Here's how the part is built. I have some questions about the finished solid (model axes, mm). A direction names the side the tool comes from. Coordinates: 2 decimals unless noted, no trailing zeros. Write each loop counter-clockwise with the first axis right and the second up, starting at its lowest first coordinate (ties: lowest second). Pieces come first, ordered by that corner, then holes. Notation, with made-up numbers: (84, 31.5) -> (95, 31.5) arc R23 cw to (95, 53.5) -> close; hole circle Ø5 at (-30.75, 50.25). An arc over 180 degrees is marked (long way). Answer in a Markdown table with one row per item. Add a question column.
from build123d import *

# Parameters (mm, degrees)
CROQUIS1_R                   = 50
SALIENTE_EXTRUIR1_DEPTH      = 120
CORTAR_EXTRUIR1_REACH        = 141.284
CROQUIS2_R                   = 45
SALIENTE_EXTRUIR2_REACH      = 141.284
SALIENTE_EXTRUIR2_END_RADIUS = 45
CROQUIS4_W                   = 47
CROQUIS4_H                   = 42
CROQUIS5_W                   = 47
CROQUIS5_H                   = 42
CORTAR_EXTRUIR2_DEPTH        = 14
CORTAR_EXTRUIR3_REACH        = 141.284


with BuildPart() as part:
    # Croquis1 → Saliente-Extruir1 (new body)
    with BuildSketch(Plane(origin=(0, 0, 0), x_dir=(1, 0, 0), z_dir=(0, 1, 0))):
        with Locations(Location((0, 0, 0), (0, 0, 270))):
            Circle(CROQUIS1_R)
    extrude(amount=SALIENTE_EXTRUIR1_DEPTH)

    # Croquis2 → Cortar-Extruir1 (cut, up to next)
    with BuildSketch(Plane(origin=(0, 120, 0), x_dir=(1, 0, 0), z_dir=(0, 1, 0)), mode=Mode.PRIVATE) as cortar_extruir1_sk1:
        with Locations(Location((0, 0, 0), (0, 0, 270))):
            Circle(CROQUIS2_R)
    cortar_extruir1_tool1 = extrude(cortar_extruir1_sk1.sketch, amount=-CORTAR_EXTRUIR1_REACH, mode=Mode.PRIVATE) & part.part
    add(cortar_extruir1_tool1.solids().sort_by_distance((0, 120, 0))[0], mode=Mode.SUBTRACT)

    # Saliente-Extruir2: up to this cylinder (the profile starts inside it)
    saliente_extruir2_end = Plane(origin=(0, 63, 0), z_dir=(0, 1, 0)) * Cylinder(SALIENTE_EXTRUIR2_END_RADIUS, 373.568, mode=Mode.PRIVATE)
    # Croquis4 → Saliente-Extruir2 (add, up to the surface)
    with BuildSketch(Plane.XY, mode=Mode.PRIVATE) as saliente_extruir2_sk1:
        with Locations((14.5, 63)):
            Rectangle(CROQUIS4_W, CROQUIS4_H)
    saliente_extruir2_tool1 = extrude(saliente_extruir2_sk1.sketch, amount=-SALIENTE_EXTRUIR2_REACH, mode=Mode.PRIVATE) & saliente_extruir2_end
    add(saliente_extruir2_tool1.solids().sort_by_distance((14.5, 63, 0))[0])

    # Croquis5 → Cortar-Extruir2 (cut)
    with BuildSketch(Plane.XY):
        with Locations((14.5, 63)):
            Rectangle(CROQUIS5_W, CROQUIS5_H)
    extrude(amount=-CORTAR_EXTRUIR2_DEPTH, mode=Mode.SUBTRACT)

    # Croquis7 → Cortar-Extruir3 (cut, up to next)
    with BuildSketch(Plane(origin=(0, 120, 0), x_dir=(1, 0, 0), z_dir=(0, 1, 0)), mode=Mode.PRIVATE) as cortar_extruir3_sk1:
        with BuildLine():
            Line((-9, -44.09081537), (-9, -49.183330509))
            ThreePointArc((-9, -49.183330509), (16.72918014, -47.118303576), (38, -32.496153619))
            Line((38, -32.496153619), (38, -24.103941586))
            ThreePointArc((38, -24.103941586), (17.61018969, -41.41112434), (-9, -44.09081537))
        make_face()
    cortar_extruir3_tool1 = extrude(cortar_extruir3_sk1.sketch, amount=-CORTAR_EXTRUIR3_REACH, mode=Mode.PRIVATE) & part.part
    add(cortar_extruir3_tool1.solids().sort_by_distance((16.242492, 120, 42.000337))[0], mode=Mode.SUBTRACT)


solid = part.part
Q1. I'm going to push flat-ended pins straight in: P1, Ø4, axis at x = 27, y = 50.5, coming from the +Z side; P2, Ø6, axis at y = 75, z = 27, coming from the -X side; P3, Ø3, axis at y = 70, z = -17, coming from the +X side; P4, Ø25, axis at x = 19.5, z = -31.5, coming from the -Y side. Where does each tip first touch, or does it pass through?
Q2. For faces 5 (the flat face through (-9, 63, -29)), 6 (the flat face through (-9, 61, 47)), 7 (the flat face through (14, 42, -29)), 8 (the flat face through (38, 61, 28)), 9 (the flat face through (14, 84, -29)), which set-ups out of +Z, -Z, +X, -X, +Y, -Y let a thin tool reach every point of the face, with its end or its side?
Q3. If we mould it in two halves opening along Z, with no side actions, what happens to faces 1 (the cylindrical face through (-14.99, 59.16, -47.7)), 2 (the flat face through (38, 63, -19)), 3 (the flat face through (14, 63, -14)), 4 (the flat face through (-7, 0, -45))? For each: pulls with the +Z half, pulls with the -Z half, needs draft (parallel to the pull), parting line crosses it, or undercut.
Q4. Imagine slicing it at D-D on x = -20. Please give me the cut outline in (y, z), plus the area to 3 significant figures.
Q5. Imagine slicing it at A-A on z = 0. Please give me the cut outline in (x, y), plus the area to 3 significant figures.
Q6. Imagine slicing it at C-C on y = 49. Please give me the cut outline in (x, z).
Q7. I need wall thicknesses on line 1 (X direction, y = 59.5, z = 0); line 2 (Z direction, x = 0, y = 39.5); line 3 (Z direction, x = 0, y = 70). Which ranges of each line are inside material? Lowest first, please. Write a range as [from, to].
Q8. Imagine slicing it at B-B on x = 0. Please give me the cut outline in (y, z).
Result sheet:
| question | item | result |
|---|---|---|
| 1 | P1 | stops at z = -14 |
| 1 | P2 | stops at x = -43.86 |
| 1 | P3 | stops at x = 47.54 |
| 1 | P4 | stops at y = 0 |
| 2 | face 5 | +Y, -Y |
| 2 | face 6 | +Z, +X, +Y, -Y |
| 2 | face 7 | +Z, -Y |
| 2 | face 8 | +Z, +Y, -Y |
| 2 | face 9 | +Z, +Y |
| 3 | face 1 | parting line crosses it |
| 3 | face 2 | undercut |
| 3 | face 3 | pulls with the +Z half |
| 3 | face 4 | needs draft |
| 4 | outline | (0, -45.83) -> (120, -45.83) -> (120, -40.31) -> (0, -40.31) -> close; (0, 40.31) -> (120, 40.31) -> (120, 45.83) -> (0, 45.83) -> close |
| 4 | area | 1,320 mm^2 |
| 5 | outline | (-50, 0) -> (-45, 0) -> (-45, 120) -> (-50, 120) -> close; (45, 0) -> (50, 0) -> (50, 120) -> (45, 120) -> close |
| 5 | area | 1,200 mm^2 |
| 6 | outline | (-9, -44.09) arc R45 cw to (-9, 44.09) -> (-9, 49.18) arc R50 ccw (long way) to (38, 32.5) -> (38, 24.1) arc R45 cw to (38, -24.1) -> (38, -14) -> (-9, -14) -> close |
| 7 | line 1 | x = [-50, -45], [45, 50] |
| 7 | line 2 | z = [-50, -45] |
| 7 | line 3 | z = [-50, -14] |
| 8 | outline | (0, -50) -> (120, -50) -> (120, -45) -> (84, -45) -> (84, -14) -> (42, -14) -> (42, -45) -> (0, -45) -> close |
